from build123d import *

# Parameters (mm, degrees)
SKETCH_1_W      = 30
SKETCH_1_H      = 15
EXTRUDE_1_DEPTH = 5
SKETCH_2_W      = 28
SKETCH_2_H      = 13
EXTRUDE_2_DEPTH = 10
FILLET_2_R      = 4
FILLET_1_R      = 5
FILLET_3_R      = 4


with BuildPart() as part:
    # Эскиз1 → Бобышка-Вытянуть1 (new body)
    with BuildSketch(Plane(origin=(0, 0, 0), x_dir=(0, 0, -1), z_dir=(1, 0, 0))):
        Rectangle(SKETCH_1_W, SKETCH_1_H)
    extrude(amount=EXTRUDE_1_DEPTH)

    # Эскиз2 → Бобышка-Вытянуть2 (add)
    with BuildSketch(Plane(origin=(5, 0, 0), x_dir=(0, 0, -1), z_dir=(1, 0, 0))):
        Rectangle(SKETCH_2_W, SKETCH_2_H)
    extrude(amount=EXTRUDE_2_DEPTH)

    # Скругление2
    fillet_2_edges = [part.edges().sort_by_distance(p)[0] for p in [
        (10, 6.5, 14),
        (10, -6.5, 14),
        (10, -6.5, -14),
        (10, 6.5, -14),
    ]]
    fillet(fillet_2_edges, radius=FILLET_2_R)

    # Скругление1
    fillet_1_edges = [part.edges().sort_by_distance(p)[0] for p in [
        (2.5, 7.5, 15),
        (2.5, 7.5, -15),
        (2.5, -7.5, -15),
        (2.5, -7.5, 15),
    ]]
    fillet(fillet_1_edges, radius=FILLET_1_R)

    # Скругление3
    fillet_3_edges = [part.edges().sort_by_distance(p)[0] for p in [
        (0, 7.5, 0),
        (0, 0, 15),
        (0, 0, -15),
        (0, -7.5, 0),
        (0, 6.035533906, 13.535533906),
        (0, -6.035533906, 13.535533906),
        (0, -6.035533906, -13.535533906),
        (0, 6.035533906, -13.535533906),
    ]]
    fillet(fillet_3_edges, radius=FILLET_3_R)


solid = part.part
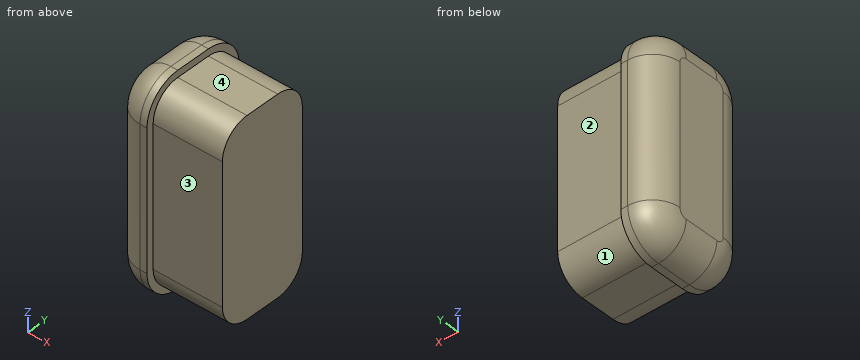
Here's how the part is built. I have some questions about the finished solid (model axes, mm). Face numbers are marked on the shaded views. A direction names the side the tool comes from. Give positions to 0.01 mm unless a question says otherwise; leave off trailing zeros. Loops run counter-clockwise (first coordinate to the right, second up) from the corner with the lowest first, then second, coordinate; pieces in that order, holes last. Notation, with made-up numbers: (4, 22) -> (24, 22) arc R14 cw to (24, 41) -> close; hole circle Ø3 at (88.5, 35.5). An arc over 180 degrees is marked (long way). Answer as a JSON object with one key per item and string values. Group by question number.
Item 1: Will these pins go through, and if not, where does the flat tip stop? pin 1 (5 mm diameter, centred on x = 13, z = -2.5, fed in from -Y); pin 2 (4 mm diameter, centred on x = 10, y = 0.5, fed in from +Z); pin 3 (8 mm diameter, centred on x = 10, z = -2.5, fed in from +Y); pin 4 (4 mm diameter, centred on y = -4.5, z = -10.5, fed in from -X).
Item 2: Imagine slicing it at B-B on y = -1. Write out the boundary of the cut face in (x, z).
Item 3: Imagine slicing it at C-C on z = 4. Write out the boundary of the cut face in (x, y).
Item 4: I need wall thicknesses on L1, parallel to Y at x = 14.25, z = 9.5; L2, parallel to Y at x = 3.75, z = 2.5; L3, parallel to Z at x = 9.5, y = -1.5. Which ranges of each line are inside material? Lowest first, please.
Item 5: On a 3-axis mill with a long thin cutter (end or side, diameter ignored), from which of +Z, -Z, +X, -X, +Y, -Y can I reach the whole of each face in a straight line? I mean the marked faces 1, 2, 3 and 4. Say none if no direction works.
Item 6: Imagine slicing it at A-A on x = 5.5. Write out the boundary of the cut face in (y, z), then the cut area to 3 significant figures.
Answer list:
{
 "1": {"pin 1": "stops at y = -6.5", "pin 2": "stops at z = 14", "pin 3": "stops at y = 6.5", "pin 4": "stops at x = 0"},
 "2": {"outline": "(0, -11) arc R4 ccw to (4, -15) -> (5, -15) -> (5, -14) -> (15, -14) -> (15, 14) -> (5, 14) -> (5, 15) -> (4, 15) arc R4 ccw to (0, 11) -> close"},
 "3": {"outline": "(0, -3.5) arc R4 ccw to (4, -7.5) -> (5, -7.5) -> (5, -6.5) -> (15, -6.5) -> (15, 6.5) -> (5, 6.5) -> (5, 7.5) -> (4, 7.5) arc R4 ccw to (0, 3.5) -> close"},
 "4": {"L1": "y = -6.5 to 6.5", "L2": "y = -7.49 to 7.49", "L3": "z = -14 to 14"},
 "5": {"face 1": "-Z, +X, +Y", "face 2": "+Z, -Z, +X, +Y", "face 3": "+Z, -Z, +X, -Y", "face 4": "+Z, +X, +Y, -Y"},
 "6": {"outline": "(-6.5, -10) arc R4 ccw to (-2.5, -14) -> (2.5, -14) arc R4 ccw to (6.5, -10) -> (6.5, 10) arc R4 ccw to (2.5, 14) -> (-2.5, 14) arc R4 ccw to (-6.5, 10) -> close", "area": "350 mm2"}
}
